Check sheet for the modelled part. Datum: model origin and axes. Units: mm. Face numbers are marked on the shaded views. A direction names the side the tool comes from. Give positions to 0.01 mm unless a question says otherwise; leave off trailing zeros. Order: outer loops, then holes, each group sorted by start corner. A loop starts at its lowest first (then second) coordinate and runs counter-clockwise, first axis right, second up.
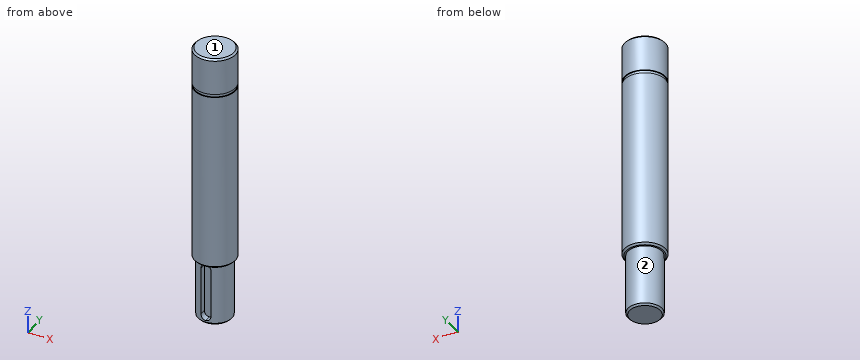
```python
from build123d import *

# Parameters (mm, degrees)
F0_R      = 5
F1_DEPTH  = 18
F2_R      = 6
F3_DEPTH  = 52.4
F4_R      = 5.75
F5_DEPTH  = 0.9
F6_R      = 6
F7_DEPTH  = 10.7
F8_SIZE2  = 0.5
F8_SIZE   = 0.5
F9_SIZE2  = 0.5
F9_SIZE   = 0.5
F10_SIZE2 = 0.5
F10_SIZE  = 0.5
F12_START = 3
F12_DEPTH = 22


with BuildPart() as f1:
    # F0 (on Top) → F1 (new body)
    with BuildSketch(Plane.XY):
        Circle(F0_R)
    extrude(amount=F1_DEPTH)

    # F2 (on face) → F3 (join)
    with BuildSketch(Plane.XY.offset(18)):
        Circle(F2_R)
    extrude(amount=F3_DEPTH)

    # F4 (on face) → F5 (join)
    with BuildSketch(Plane.XY.offset(70.4)):
        Circle(F4_R)
    extrude(amount=F5_DEPTH)

    # F6 (on face) → F7 (join)
    with BuildSketch(Plane.XY.offset(71.3)):
        Circle(F6_R)
    extrude(amount=F7_DEPTH)

    # F8
    f8_edges = [f1.edges().sort_by_distance(p)[0] for p in [
        (-6, 0, 82),
    ]]
    chamfer(f8_edges, length=F8_SIZE, length2=F8_SIZE2)

    # F9
    f9_edges = [f1.edges().sort_by_distance(p)[0] for p in [
        (-6, 0, 18),
    ]]
    chamfer(f9_edges, length=F9_SIZE, length2=F9_SIZE2)

    # F10
    f10_edges = [f1.edges().sort_by_distance(p)[0] for p in [
        (-5, 0, 0),
    ]]
    chamfer(f10_edges, length=F10_SIZE, length2=F10_SIZE2)

    # F11 (on Front) → F12 (cut)
    with BuildSketch(Plane.XZ.offset(F12_START)):
        with BuildLine():
            Line((1.5, 2.5), (1.5, 16.5))
            ThreePointArc((1.5, 16.5), (0, 18), (-1.5, 16.5))
            Line((-1.5, 16.5), (-1.5, 2.5))
            ThreePointArc((-1.5, 2.5), (-1.0606601718, 1.4393398282), (0, 1))
            ThreePointArc((0, 1), (1.0606601718, 1.4393398282), (1.5, 2.5))
        make_face()
    extrude(amount=F12_DEPTH, mode=Mode.SUBTRACT)


solid = f1.part
```
Q1. Sectioned sample at C-C, the plane z = 40.5. Record the cut outline in (x, y), plus the area to 3 significant figures.
Q2. Material ranges on line 1 (Z direction, x = -4.25, y = -4); line 2 (Y direction, x = -4.25, z = 61.5); line 3 (X direction, y = -3.25, z = 6), recorded low to high.
Q3. Go/stop test with flat-tipped pins: P1, Ø3, axis at x = -4, z = 37.5, coming from the +Y side; P2, Ø1.5, axis at y = -4, z = 58.5, coming from the -X side; P3, Ø4, axis at x = 3, z = 24, coming from the -Y side. Record where each tip stops, or that it passes through.
Q4. Tool access check on the marked faces 1 and 2. Record the directions out of +Z, -Z, +X, -X, +Y, -Y that give a thin tool (end or side, any length) a straight path to the whole face; none if there is none.
Q5. Sectioned sample at A-A, the plane y = 0. Record the cut outline in (x, z), plus the area to 3 significant figures.
Q6. Sectioned sample at B-B, the plane z = 10. Record the cut outline in (x, y), plus the area to 3 significant figures.
Filled in:
1. outline: circle Ø12 at (0, 0)
1. area: 113 mm2
2. line 1: z = 18.34 to 70.4, 71.3 to 81.66
2. line 2: y = -4.24 to 4.24
2. line 3: x = -3.8 to -1.5, 1.5 to 3.8
3. P1: stops at y = 5.45
3. P2: stops at x = -5.04
3. P3: stops at y = -5.92
4. face 1: +Z, +X, -X, +Y, -Y
4. face 2: -Z
5. outline: (-6, 18.5) - (-5.5, 18) - (-5, 18) - (-5, 0.5) - (-4.5, 0) - (4.5, 0) - (5, 0.5) - (5, 18) - (5.5, 18) - (6, 18.5) - (6, 70.4) - (5.75, 70.4) - (5.75, 71.3) - (6, 71.3) - (6, 81.5) - (5.5, 82) - (-5.5, 82) - (-6, 81.5) - (-6, 71.3) - (-5.75, 71.3) - (-5.75, 70.4) - (-6, 70.4) - close
5. area: 947 mm2
6. outline: (-1.5, -4.77) - (-1.5, -3) - (1.5, -3) - (1.5, -4.77) arc R5 ccw (long way) to start
6. area: 72.8 mm2
